```python
from build123d import *

# Parameters (mm, degrees)
F1_DEPTH = 42.5
F2_R     = 2.75
F3_DEPTH = 5.001


with BuildPart() as f1:
    # F0 (on Front) → F1 (new body, symmetric)
    with BuildSketch(Plane.XZ):
        with BuildLine():
            Line((81.504221, 1.853635), (81.504221, 26.353635))
            ThreePointArc((81.504221, 26.353635), (80.771988, 28.121402), (79.004221, 28.853635))
            ThreePointArc((79.004221, 28.853635), (77.236454, 28.121402), (76.504221, 26.353635))
            Line((76.504221, 26.353635), (76.504221, 6.853635))
            ThreePointArc((76.504221, 6.853635), (75.625541, 4.732315), (73.504221, 3.853635))
            Line((73.504221, 3.853635), (19.504221, 3.853635))
            ThreePointArc((19.504221, 3.853635), (17.382901, 4.732315), (16.504221, 6.853635))
            Line((16.504221, 6.853635), (16.504221, 52.853635))
            ThreePointArc((16.504221, 52.853635), (15.625541, 54.974956), (13.504221, 55.853635))
            Line((13.504221, 55.853635), (-30.495779, 55.853635))
            ThreePointArc((-30.495779, 55.853635), (-32.617099, 54.974956), (-33.495779, 52.853635))
            Line((-33.495779, 52.853635), (-33.495779, 28.353635))
            ThreePointArc((-33.495779, 28.353635), (-32.763546, 26.585868), (-30.995779, 25.853635))
            ThreePointArc((-30.995779, 25.853635), (-29.228012, 26.585868), (-28.495779, 28.353635))
            Line((-28.495779, 28.353635), (-28.495779, 47.853635))
            ThreePointArc((-28.495779, 47.853635), (-27.617099, 49.974956), (-25.495779, 50.853635))
            Line((-25.495779, 50.853635), (8.504221, 50.853635))
            ThreePointArc((8.504221, 50.853635), (10.625541, 49.974956), (11.504221, 47.853635))
            Line((11.504221, 47.853635), (11.504221, 11.853635))
            ThreePointArc((11.504221, 11.853635), (11.211328, 11.146529), (10.504221, 10.853635))
            Line((10.504221, 10.853635), (8.504221, 10.853635))
            Line((8.504221, 10.853635), (11.504221, 1.853635))
            ThreePointArc((11.504221, 1.853635), (12.382901, -0.267685), (14.504221, -1.146365))
            Line((14.504221, -1.146365), (78.504221, -1.146365))
            ThreePointArc((78.504221, -1.146365), (80.625541, -0.267685), (81.504221, 1.853635))
        make_face()
    extrude(amount=F1_DEPTH, both=True)

    # F2 (on face) → F3 (cut, through all)
    with BuildSketch(Plane.XY.offset(3.853635)):
        with Locations((36.504221, -22.5)):
            Circle(F2_R)
        with Locations((56.504221, -22.5)):
            Circle(F2_R)
    extrude(amount=-F3_DEPTH, mode=Mode.SUBTRACT)


solid = f1.part
```
Could you check a few things on this model? Use its own coordinates, in mm. A direction names the side the tool comes from. Give positions to 0.01 mm unless a question says otherwise; leave off trailing zeros. Loops run counter-clockwise (first coordinate to the right, second up) from the corner with the lowest first, then second, coordinate; pieces in that order, holes last. Notation, with made-up numbers: (0.25, 69) - (21.25, 69) arc R28 ccw to (21.25, 93) - close; hole circle Ø10 at (61.25, -13). An arc over 180 degrees is marked (long way). Answer in a Markdown table with one row per item. Add a question column.
Q1. If we section it at D-D (x = 46.5): List the corners of the cut face in (y, z) for me.
Q2. Please list where these lines run through material, in increasing order: L1, parallel to X at y = 4, z = 46; L2, parallel to X at y = -22, z = 0; L3, parallel to X at y = -21.5, z = 24. Write a range as from..to.
Q3. We'd pull the mould along X, two halves only. Please class faces 4 (the face through (-32.59, -0.59, 55)), 5 (the face through (15, -42.5, 25)), 6 (the face through (16.504, -1, 30)), 7 (the face through (17.406, -0.595, 4.709)): +X half, -X half, draft (parallel to the pull), parting line (faces both ways), or undercut.
Q4. If we section it at B-B (z = 21): List the corners of the cut face in (x, y) for me, plus the area to 3 significant figures.
Q5. If we section it at A-A (y = -22.5): State how many separate pieces and enclosed holes the cut face has, plus the area to 3 significant figures.
Q6. For pin 1 (12 mm diameter, centred on x = -5, z = 43, fed in from -Y); pin 2 (10 mm diameter, centred on y = -27, z = 43.5, fed in from +X); pin 3 (21.5 mm diameter, centred on y = -1, z = 35, fed in from +X), each with a flat end and sliding along its axis, tell me the tip position at first contact or that it passes through.
Q7. If we section it at C-C (y = 1.5): List the corners of the cut face in (x, z) for me.
Q8. Which directions (+Z, -Z, +X, -X, +Y, -Y) give clear straight access to the entire face, cutting with the end or side of a thin tool? Please do faces 1 (the face through (46, -1, -1.146)), 2 (the face through (76.504, -1, 17)), 3 (the face through (-9, -1, 50.854)).
The answers:
| question | item | result |
|---|---|---|
| 1 | outline | (-42.5, -1.15) - (42.5, -1.15) - (42.5, 3.85) - (-42.5, 3.85) - close |
| 2 | L1 | x = -33.5..-28.5, 11.5..16.5 |
| 2 | L2 | x = 12.15..33.8, 39.21..53.8, 59.21..80.86 |
| 2 | L3 | x = 11.5..16.5, 76.5..81.5 |
| 3 | face 4 | -X half |
| 3 | face 5 | draft |
| 3 | face 6 | undercut |
| 3 | face 7 | undercut |
| 4 | outline | (11.5, -42.5) - (16.5, -42.5) - (16.5, 42.5) - (11.5, 42.5) - close; (76.5, -42.5) - (81.5, -42.5) - (81.5, 42.5) - (76.5, 42.5) - close |
| 4 | area | 850 mm^2 |
| 5 | separate pieces | 3 |
| 5 | enclosed holes | 0 |
| 5 | area | 1,040 mm^2 |
| 6 | pin 1 | passes through |
| 6 | pin 2 | stops at x = 16.5 |
| 6 | pin 3 | stops at x = 81.5 |
| 7 | outline | (-33.5, 28.35) arc R2.5 ccw to (-28.5, 28.35) - (-28.5, 47.85) arc R3 cw to (-25.5, 50.85) - (8.5, 50.85) arc R3 cw to (11.5, 47.85) - (11.5, 11.85) arc R1 cw to (10.5, 10.85) - (8.5, 10.85) - (11.5, 1.85) arc R3 ccw to (14.5, -1.15) - (78.5, -1.15) arc R3 ccw to (81.5, 1.85) - (81.5, 26.35) arc R2.5 ccw to (76.5, 26.35) - (76.5, 6.85) arc R3 cw to (73.5, 3.85) - (19.5, 3.85) arc R3 cw to (16.5, 6.85) - (16.5, 52.85) arc R3 ccw to (13.5, 55.85) - (-30.5, 55.85) arc R3 ccw to (-33.5, 52.85) - close |
| 8 | face 1 | -Z, +X, -X, +Y, -Y |
| 8 | face 2 | +Z, +Y, -Y |
| 8 | face 3 | -Z, +Y, -Y |
